from build123d import *

# Parameters (mm, degrees)
SKETCH_W        = 29
SKETCH_H        = 47
PAD_DEPTH       = 40
SKETCH001_R     = 9.75
PAD001_DEPTH    = 10
SKETCH002_W     = 56
SKETCH002_H     = 6
POCKET_DEPTH    = 100
SKETCH003_W     = 54.44
SKETCH003_H     = 5.76
POCKET001_DEPTH = 40.001
SKETCH004_R     = 1.1
SKETCH004_R_2   = 1
POCKET002_DEPTH = 5
SKETCH005_W     = 54.27
SKETCH005_H     = 70.91
POCKET003_DEPTH = 50.001


with BuildPart() as part:
    # Sketch → Pad (new body)
    with BuildSketch(Plane.XY.offset(10)):
        with BuildLine():
            Line((0, 0), (40, 0))
            Line((40, 0), (40, 60))
            ThreePointArc((40, 60), (20, 68.990653), (0, 60))
            Line((0, 60), (0, 0))
        make_face()
        with Locations((20, 30)):
            Rectangle(SKETCH_W, SKETCH_H, mode=Mode.SUBTRACT)
    extrude(amount=PAD_DEPTH)

    # Sketch001 (on Face9 of Pad) → Pad001 (join)
    with BuildSketch(Plane(origin=(0, 0, 10), x_dir=(1, 0, 0), z_dir=(0, 0, -1))):
        with BuildLine():
            Line((40, -60), (40, 30))
            ThreePointArc((40, 30), (20, 50), (0, 30))
            Line((0, 30), (0, -60))
            ThreePointArc((0, -60), (20, -68.990653), (40, -60))
        make_face()
        with Locations((20, -42.25)):
            Circle(SKETCH001_R, mode=Mode.SUBTRACT)
    extrude(amount=PAD001_DEPTH)

    # Sketch002 (on Face7 of Pad001) → Pocket (cut)
    with BuildSketch(Plane(origin=(0, 0, 0), x_dir=(0, -1, 0), z_dir=(-1, 0, 0))):
        with Locations((-48, 3)):
            Rectangle(SKETCH002_W, SKETCH002_H)
    extrude(amount=-POCKET_DEPTH, mode=Mode.SUBTRACT)

    # Sketch003 (on Face8 of Pocket) → Pocket001 (cut, through all)
    with BuildSketch(Plane.YZ.offset(40)):
        with Locations((-27.22, 7.88)):
            Rectangle(SKETCH003_W, SKETCH003_H)
    extrude(amount=-POCKET001_DEPTH, mode=Mode.SUBTRACT)

    # Sketch004 (on Face12 of Pocket001) → Pocket002 (cut)
    with BuildSketch(Plane(origin=(0, 0, 0), x_dir=(1, 0, 0), z_dir=(0, 0, -1))):
        with Locations((11.98, 30)):
            Circle(SKETCH004_R)
        with Locations((14.34, 35.7)):
            Circle(SKETCH004_R_2)
        with Locations((20, 37.98)):
            Circle(SKETCH004_R)
        with Locations((25.66, 35.7)):
            Circle(SKETCH004_R_2)
        with Locations((28.02, 30)):
            Circle(SKETCH004_R)
        with Locations((25.66, 24.34)):
            Circle(SKETCH004_R_2)
        with Locations((20, 22.02)):
            Circle(SKETCH004_R)
        with Locations((14.34, 24.34)):
            Circle(SKETCH004_R_2)
    extrude(amount=-POCKET002_DEPTH, mode=Mode.SUBTRACT)

    # Sketch005 (on Face12 of Pocket002) → Pocket003 (cut, through all)
    with BuildSketch(Plane(origin=(0, 0, 0), x_dir=(1, 0, 0), z_dir=(0, 0, -1))):
        with Locations((27.135, -35.455)):
            Rectangle(SKETCH005_W, SKETCH005_H)
    extrude(amount=-POCKET003_DEPTH, mode=Mode.SUBTRACT)


solid = part.part
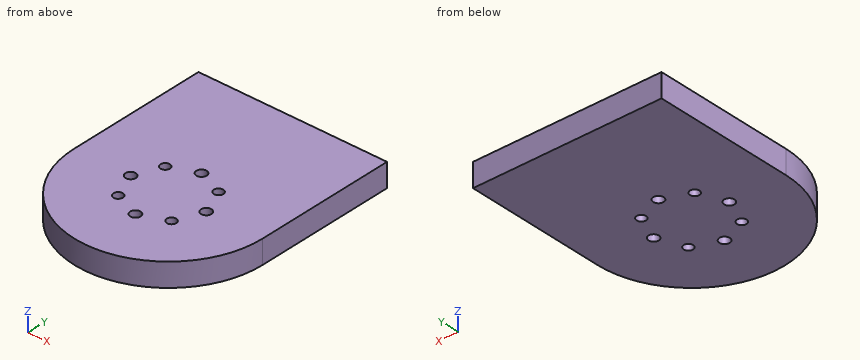
Here's how the part is built. I have some questions about the finished solid (model axes, mm). Coordinates: 2 decimals unless noted, no trailing zeros. Loops run counter-clockwise (first coordinate to the right, second up) from the corner with the lowest first, then second, coordinate; pieces in that order, holes last.
1. Imagine slicing it at B-B, the plane x = 28.02. Please give me the cut outline in (y, z).
2. For P1, Ø1.2, axis at x = 14.34, y = -24.34, coming from the -Z side; P2, Ø2.5, axis at x = 25.66, y = -35.7, coming from the +Z side; P3, Ø1.5, axis at y = -37, z = 3, coming from the +X side, each with a flat end and sliding along its axis, tell me the tip position at first contact or that it passes through.
3. Imagine slicing it at C-C, the plane z = 2.2. Count the separate pieces of the cut face and the enclosed holes in it, and give its area (3 significant figures).
4. Imagine slicing it at D-D, the plane x = 6.5. Please give me the cut outline in (y, z), and give its area (3 significant figures).
5. Imagine slicing it at A-A, the plane y = -22.02. Please give me the cut outline in (x, z).
6. I need wall thicknesses on L1, parallel to X at y = -30, z = 1.6; L2, parallel to Y at x = 20, z = 1.1; L3, parallel to X at y = -22, z = 3.7. Which ranges of each line are inside material? Lowest first, please.
Taken from the geometry:
1. outline: (-48.32, 0) - (-31.1, 0) - (-31.1, 5) - (-48.32, 5) - close; (-28.9, 0) - (0, 0) - (0, 5) - (-28.9, 5) - close
2. P1: passes through
2. P2: stops at z = 5
2. P3: stops at x = 39
3. separate pieces: 1
3. enclosed holes: 8
3. area: 1,800 mm2
4. outline: (-44.76, 0) - (0, 0) - (0, 5) - (-44.76, 5) - close
4. area: 224 mm2
5. outline: (0, 0) - (18.9, 0) - (18.9, 5) - (0, 5) - close; (21.1, 0) - (40, 0) - (40, 5) - (21.1, 5) - close
6. L1: x = 0 to 10.88, 13.08 to 26.92, 29.12 to 40
6. L2: y = -50 to -39.08, -36.88 to -23.12, -20.92 to 0
6. L3: x = 0 to 18.9, 21.1 to 40
